Geometry: final body of the model. Coordinates: model frame, mm. A direction names the side the tool comes from. Give positions to 0.01 mm unless a question says otherwise; leave off trailing zeros. Loops run counter-clockwise (first coordinate to the right, second up) from the corner with the lowest first, then second, coordinate; pieces in that order, holes last. Notation, with made-up numbers: M 35,0.5 L 52,0.5 A28 cw 52,39.5 Z; hole C 46.25,74 d10. An arc over 180 degrees is marked long. Put each result on its own line as item: value.
```python
from build123d import *

# Parameters (mm, degrees)
BASE_FLANGE1_DEPTH = 12.7
SKETCH2_R          = 24.60625
SKETCH2_R_2        = 8.3312
CUT_EXTRUDE1_DEPTH = 196.159220654
CUT_EXTRUDE2_DEPTH = 196.159220654
FILLET1_R          = 3.175
SKETCH8_W          = 7.14375
SKETCH8_H          = 25.4
CUT_EXTRUDE3_DEPTH = 195.449637912
FILLET2_R          = 0.79375


# Sheet-metal steps are written as plain solids
with BuildPart() as part:
    # Sketch1 → Base-Flange1 (new body)
    with BuildSketch(Plane(origin=(0, 0, 0), x_dir=(1, 0, 0), z_dir=(0, 1, 0))):
        with BuildLine():
            Line((-95.25, 0), (95.25, 0))
            Line((95.25, 0), (39.960205447, -142.504060335))
            ThreePointArc((39.960205447, -142.504060335), (0, -169.8625), (-39.960205447, -142.504060335))
            Line((-39.960205447, -142.504060335), (-95.25, 0))
        make_face()
    extrude(amount=-BASE_FLANGE1_DEPTH)

    # Sketch2 → Cut-Extrude1 (cut, through all)
    with BuildSketch(Plane(origin=(0, 0, 0), x_dir=(1, 0, 0), z_dir=(0, 1, 0))):
        with Locations(Location((0, -127, 0), (0, 0, 270))):
            Circle(SKETCH2_R)
        with Locations(Location((-25.4, -76.2, 0), (0, 0, 270))):
            Circle(SKETCH2_R_2)
        with Locations(Location((25.4, -76.2, 0), (0, 0, 270))):
            Circle(SKETCH2_R_2)
    extrude(amount=-CUT_EXTRUDE1_DEPTH, mode=Mode.SUBTRACT)

    # Sketch7 → Cut-Extrude2 (cut, through all)
    with BuildSketch(Plane(origin=(0, 0, 0), x_dir=(1, 0, 0), z_dir=(0, 1, 0))):
        with BuildLine():
            Line((53.975, -25.4), (28.575, -25.4))
            ThreePointArc((28.575, -25.4), (22.225, -19.05), (28.575, -12.7))
            Line((28.575, -12.7), (53.975, -12.7))
            ThreePointArc((53.975, -12.7), (60.325, -19.05), (53.975, -25.4))
        make_face()
        with BuildLine():
            Line((-28.575, -25.4), (-53.975, -25.4))
            ThreePointArc((-53.975, -25.4), (-60.325, -19.05), (-53.975, -12.7))
            Line((-53.975, -12.7), (-28.575, -12.7))
            ThreePointArc((-28.575, -12.7), (-22.225, -19.05), (-28.575, -25.4))
        make_face()
    extrude(amount=-CUT_EXTRUDE2_DEPTH, mode=Mode.SUBTRACT)

    # Fillet1
    fillet1_edges = [part.edges().sort_by_distance(p)[0] for p in [
        (-95.25, -6.35, 0),
        (95.25, -6.35, 0),
    ]]
    fillet(fillet1_edges, radius=FILLET1_R)

    # Sketch8 → Cut-Extrude3 (cut, through all)
    with BuildSketch(Plane(origin=(0, 0, 0), x_dir=(1, 0, 0), z_dir=(0, 1, 0))):
        with Locations((44.846875, -63.5)):
            Rectangle(SKETCH8_W, SKETCH8_H)
        with Locations((-44.846875, -63.5)):
            Rectangle(SKETCH8_W, SKETCH8_H)
    extrude(amount=-CUT_EXTRUDE3_DEPTH, mode=Mode.SUBTRACT)

    # Fillet2
    fillet2_edges = [part.edges().sort_by_distance(p)[0] for p in [
        (41.275, -6.35, 76.2),
        (41.275, -6.35, 50.8),
        (48.41875, -6.35, 50.8),
        (48.41875, -6.35, 76.2),
        (-48.41875, -6.35, 76.2),
        (-48.41875, -6.35, 50.8),
        (-41.275, -6.35, 50.8),
        (-41.275, -6.35, 76.2),
    ]]
    fillet(fillet2_edges, radius=FILLET2_R)


solid = part.part
```
Item 1: Mould query, pull axis Z, two halves, no side actions, for faces 3 (the cylindrical face through (93.21, -6.44, 1.35)), 4 (the cylindrical face through (-22.227, -6.261, 18.91)), 5 (the cylindrical face through (0.72, -6.261, 169.856)). Classes: pulls with the +Z half, pulls with the -Z half, needs draft (parallel to the pull), parting line crosses it, or undercut.
Output values:
face 3: parting line crosses it
face 4: undercut
face 5: pulls with the +Z half
Item 2: Section A-A on x = 0. Output: boundary loops of the cut face in (y, z), then the cut area to 3 significant figures.
Output values:
outline: M -12.7,0 L 0,0 L 0,102.39 L -12.7,102.39 Z; M -12.7,151.61 L 0,151.61 L 0,169.86 L -12.7,169.86 Z
area: 1,530 mm²
Item 3: Line query: probe 1 along Z at (x, y) = (-18.5, -8.75); probe 2 along X at (y, z) = (-6.75, 18); probe 3 along Z at (x, y) = (36, -8.5). Output: solid intervals per line, ascending. Write a range as [from, to].
Output values:
probe 1: [0, 71.53], [80.87, 110.78], [143.22, 165.66]
probe 2: [-88.27, -60.24], [-22.31, 22.31], [60.24, 88.27]
probe 3: [0, 12.7], [25.4, 150.26]
Item 4: Section B-B on y = -7.5. Count the separate pieces of the cut face and the enclosed holes in it, then the cut area to 3 significant figures.
Output values:
separate pieces: 1
enclosed holes: 7
area: 17,200 mm²
Item 5: Pin query (flat end, axial travel): pin 1 Ø6.5 at (y, z) = (-7, 58) entering from -X; pin 2 Ø1.5 at (y, z) = (-6, 32) entering from -X; pin 3 Ø6 at (y, z) = (-6, 152.5) entering from +X. Return the tip coordinate at first contact, or that it passes through.
Output values:
pin 1: x = -74.01
pin 2: x = -83.13
pin 3: x = 36.48
Item 6: Set-up query: faces 1 (the flat face through (67.14, -6.26, 72.45)), 2 (the flat face through (-41, -6, 12.7)). Return all of +Z, -Z, +X, -X, +Y, -Y with unobstructed straight access to the full face (end or side cutting, diameter ignored); none if empty.
Output values:
face 1: +Z, +X, +Y, -Y
face 2: +Y, -Y
Item 7: Section C-C on z = 127. Output: boundary loops of the cut face in (x, y), then the cut area to 3 significant figures.
Output values:
outline: M -45.98,-12.7 L -24.61,-12.7 L -24.61,0 L -45.98,0 Z; M 24.61,-12.7 L 45.98,-12.7 L 45.98,0 L 24.61,0 Z
area: 543 mm²
Item 8: Section D-D on z = 19.05. Output: boundary loops of the cut face in (x, y) (3 decimals), then the cut area to 3 significant figures.
Output values:
outline: M -87.859,-12.7 L -60.325,-12.7 L -60.325,0 L -87.859,0 Z; M -22.225,-12.7 L 22.225,-12.7 L 22.225,0 L -22.225,0 Z; M 60.325,-12.7 L 87.859,-12.7 L 87.859,0 L 60.325,0 Z
area: 1,260 mm²
